Input: part model. Units: mm. Frame: model coordinates. Face numbers are marked on the shaded views. A direction names the side the tool comes from. Round coordinates to 2 decimals unless told otherwise and drop trailing zeros. Loops run counter-clockwise (first coordinate to the right, second up) from the corner with the lowest first, then second, coordinate; pieces in that order, holes last.
1) First-contact query: pin 1 (1.5 mm diameter, centred on x = 5, z = 10.5, fed in from -Y); pin 2 (10 mm diameter, centred on y = 116, z = -6.5, fed in from -X); pin 3 (1 mm diameter, centred on y = 25.5, z = -3, fed in from +X). Flat tips, straight axial feed; report the tip coordinate or a pass-through.
2) Ray query, line 1 along Y through (x, z) = (13, -7); line 2 along Z through (x, y) = (0.25, 61). Return the intervals inside material, ascending.
3) Access query for the marked faces 1, 2 and 3. Directions: +Z, -Z, +X, -X, +Y, -Y. A direction counts if a zero-diameter tool reaches every point of the face in a straight line with its end or side. Return the directions, or none.
4) Section B-B, the plane y = 63. Return loops of the section in (x, z).
5) Section A-A, the plane z = 0. Return loops of the section in (x, y), and give its area (3 significant figures).
from build123d import *

# Parameters (mm, degrees)
SKETCH1_R           = 15
BOSS_EXTRUDE1_DEPTH = 15
SKETCH2_R           = 10
BOSS_EXTRUDE2_DEPTH = 133.5
SKETCH4_R           = 7.5
BOSS_EXTRUDE3_DEPTH = 15


# Read off the part's stored shape, not the designer's step: M12x1.5 Machine Threads Stud1
with BuildPart() as part:
    # Sketch1 → Boss-Extrude1 (new body)
    with BuildSketch(Plane(origin=(0, 0, 0), x_dir=(1, 0, 0), z_dir=(0, 1, 0))):
        with Locations(Location((0, 0, 0), (0, 0, 270))):
            Circle(SKETCH1_R)
    extrude(amount=BOSS_EXTRUDE1_DEPTH)

    # Sketch2 → Boss-Extrude2 (add)
    with BuildSketch(Plane(origin=(0, 15, 0), x_dir=(1, 0, 0), z_dir=(0, 1, 0))):
        with Locations(Location((0, 0, 0), (0, 0, 270))):
            Circle(SKETCH2_R)
    extrude(amount=BOSS_EXTRUDE2_DEPTH)

    # Sketch4 → Boss-Extrude3 (add)
    with BuildSketch(Plane.XZ):
        with Locations(Location((0, 0, 0), (0, 0, 270))):
            Circle(SKETCH4_R)
    extrude(amount=BOSS_EXTRUDE3_DEPTH)

    # M12x1.5 Machine Threads Stud1 outline → M12x1.5 Machine Threads Stud1 (revolve, cut)
    with BuildSketch(Plane.XY):
        Polygon((7.5, 0), (6, 0), (6, -14.172), (5.172, -15), (7.5, -15), align=None)
    revolve(axis=Axis((0, 0, 0), (0, 1, 0)), mode=Mode.SUBTRACT)


solid = part.part
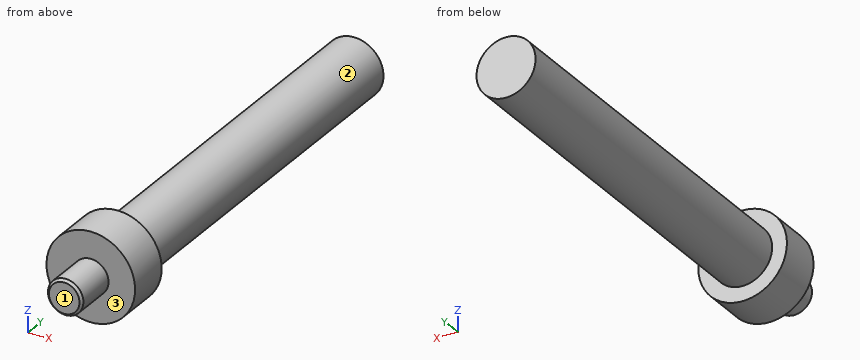
Final values:
1. pin 1: stops at y = 0
1. pin 2: stops at x = -9.89
1. pin 3: stops at x = 9.68
2. line 1: y = 0 to 15
2. line 2: z = -10 to 10
3. face 1: +Z, -Z, +X, -X, -Y
3. face 2: +Y
3. face 3: -Y
4. outline: circle Ø20 at (0, 0)
5. outline: (-15, 0) - (-6, 0) - (-6, -14.17) - (-5.17, -15) - (5.17, -15) - (6, -14.17) - (6, 0) - (15, 0) - (15, 15) - (10, 15) - (10, 148.5) - (-10, 148.5) - (-10, 15) - (-15, 15) - close
5. area: 3,300 mm2
